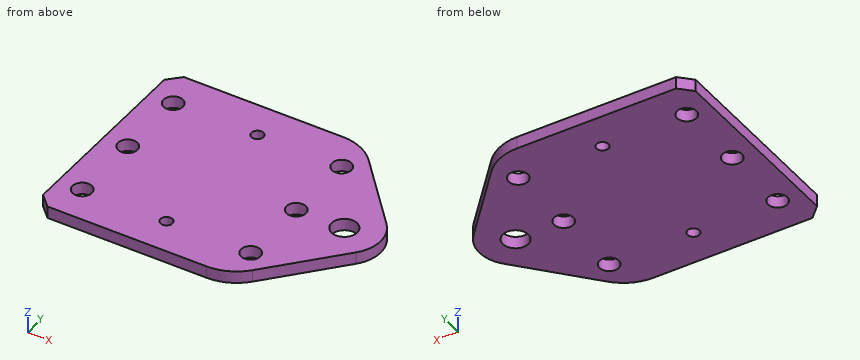
from build123d import *

# Parameters (mm, degrees)
SKETCH1_R              = 3.3782
BOSS_EXTRUDE1_DEPTH    = 3.175
F_10_CLEARANCE_HOLE1_D = 5.1054
CHAMFER1_SIZE          = 3.175
SKETCH4_R              = 1.5875
CUT_EXTRUDE1_DEPTH     = 4.175


with BuildPart() as part:
    # Sketch1 → Boss-Extrude1 (new body)
    with BuildSketch(Plane.XY):
        with BuildLine():
            Line((0, 0), (45.105286642, 0))
            ThreePointArc((45.105286642, 0), (50.301519782, 1.111679969), (54.588060278, 4.252100606))
            Line((54.588060278, 4.252100606), (70.612080227, 22.239075455))
            ThreePointArc((70.612080227, 22.239075455), (73.025, 28.575), (70.612080227, 34.910924545))
            Line((70.612080227, 34.910924545), (54.588060278, 52.897899394))
            ThreePointArc((54.588060278, 52.897899394), (50.301519782, 56.038320031), (45.105286642, 57.15))
            Line((45.105286642, 57.15), (0, 57.15))
            Line((0, 57.15), (0, 0))
        make_face()
        with Locations((63.5, 28.575)):
            Circle(SKETCH1_R, mode=Mode.SUBTRACT)
    extrude(amount=BOSS_EXTRUDE1_DEPTH)

    # #10 Clearance Hole1 (through all)
    with Locations(Plane.XY.offset(3.175)):
        with Locations((50.8, 28.575), (6.35, 28.575), (6.35, 47.625), (50.8, 47.625), (50.8, 9.525), (6.35, 9.525)):
            Hole(F_10_CLEARANCE_HOLE1_D / 2)

    # Chamfer1
    chamfer1_edges = [part.edges().sort_by_distance(p)[0] for p in [
        (0, 57.15, 1.5875),
        (0, 0, 1.5875),
    ]]
    chamfer(chamfer1_edges, length=CHAMFER1_SIZE)

    # Sketch4 → Cut-Extrude1 (cut, through all)
    with BuildSketch(Plane.XY.offset(3.175)):
        with Locations((28.575, 47.625)):
            Circle(SKETCH4_R)
        with Locations((28.575, 9.525)):
            Circle(SKETCH4_R)
    extrude(amount=-CUT_EXTRUDE1_DEPTH, mode=Mode.SUBTRACT)


solid = part.part
Source: CAD feature listing. Evaluate the final solid. Frame: model axes, mm. Round coordinates to 2 decimals unless told otherwise and drop trailing zeros. Loops run counter-clockwise (first coordinate to the right, second up) from the corner with the lowest first, then second, coordinate; pieces in that order, holes last. Notation, with made-up numbers: (-36, 85.25) - (-23, 85.25) arc R20 cw to (-23, 96.25) - close; hole circle Ø8 at (84, 25). An arc over 180 degrees is marked (long way). Write item = value, one per line. Start each with the question number.
Item 1: First-contact query: pin 1 Ø6 at (x, y) = (50.8, 28.575) entering from +Z (3 decimals); pin 2 Ø1 at (x, z) = (52.5, 2.5) entering from -Y. Flat tips, straight axial feed; report the tip coordinate or a pass-through.
Item 2: Section query B-B on x = 63.5. Output: boundary loops of the cut face in (y, z) (3 decimals), plus the area to 3 significant figures.
Item 3: Section query D-D on x = 50.8. Output: boundary loops of the cut face in (y, z) (3 decimals).
Item 4: Material intervals for line 1 (Y direction, x = 50.8, z = 1.65); line 2 (Y direction, x = 30, z = 2.25); line 3 (X direction, y = 9, z = 1), sorted ascending.
Item 5: Section query A-A on x = 6.35. Output: boundary loops of the cut face in (y, z) (3 decimals), plus the area to 3 significant figures.
Item 6: Section query C-C on z = 1.6. Count the separate pieces of the cut face and the enclosed holes in it, plus the area to 3 significant figures.
Results list:
q1.pin_1 = 3.175
q1.pin_2 = 2.03
q2.outline = (14.256, 0) - (25.197, 0) - (25.197, 3.175) - (14.256, 3.175) - close; (31.953, 0) - (42.894, 0) - (42.894, 3.175) - (31.953, 3.175) - close
q2.area = 69.5 mm²
q3.outline = (1.348, 0) - (6.972, 0) - (6.972, 3.175) - (1.348, 3.175) - close; (12.078, 0) - (26.022, 0) - (26.022, 3.175) - (12.078, 3.175) - close; (31.128, 0) - (45.072, 0) - (45.072, 3.175) - (31.128, 3.175) - close; (50.178, 0) - (55.802, 0) - (55.802, 3.175) - (50.178, 3.175) - close
q4.line_1 = 1.35 to 6.97, 12.08 to 26.02, 31.13 to 45.07, 50.18 to 55.8
q4.line_2 = 0 to 8.83, 10.22 to 46.93, 48.32 to 57.15
q4.line_3 = 0 to 3.85, 8.85 to 27.08, 30.07 to 48.3, 53.3 to 58.82
q5.outline = (0, 0) - (6.972, 0) - (6.972, 3.175) - (0, 3.175) - close; (12.078, 0) - (26.022, 0) - (26.022, 3.175) - (12.078, 3.175) - close; (31.128, 0) - (45.072, 0) - (45.072, 3.175) - (31.128, 3.175) - close; (50.178, 0) - (57.15, 0) - (57.15, 3.175) - (50.178, 3.175) - close
q5.area = 133 mm²
q6.separate_pieces = 1
q6.enclosed_holes = 9
q6.area = 3,420 mm²
